Geometry: final body of the model. Coordinates: model frame, mm. Round coordinates to 2 decimals unless told otherwise and drop trailing zeros. Order: outer loops, then holes, each group sorted by start corner. A loop starts at its lowest first (then second) coordinate and runs counter-clockwise, first axis right, second up. Notation, with made-up numbers: (45, -13.75) -> (99, -13.75) arc R31 cw to (99, 12.25) -> close; hole circle Ø6 at (15.5, 54). An arc over 180 degrees is marked (long way). Put each result on its own line as item: value.
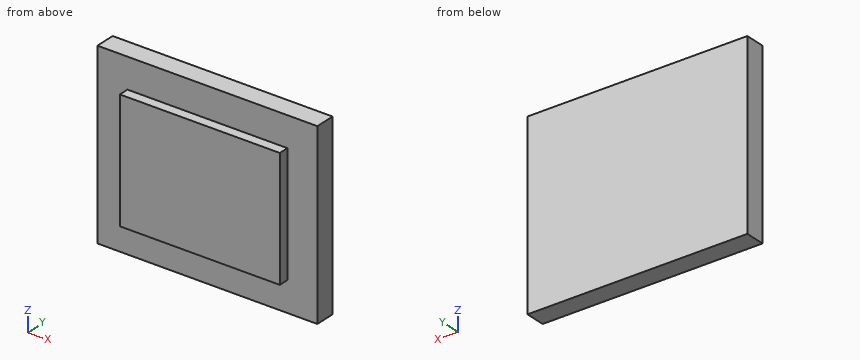
Solid Edge part; units mm, degrees
sketch "Sketch1" plane through (0, 0, 0) normal (0, -1, 0) x (1, 0, 0)
  line L0 (139.7, 114.3) -> (-139.7, 114.3)
  line L1 (-139.7, 114.3) -> (-139.7, -114.3)
  line L2 (-139.7, -114.3) -> (139.7, -114.3)
  line L3 (139.7, -114.3) -> (139.7, 114.3)
extrude "Protrusion1" add sketch "Sketch1" against normal blind 25.4
sketch "Sketch2" plane through (0, 0, 0) normal (0, -1, 0) x (1, 0, 0)
  line L0 (101.6, 76.2) -> (-101.6, 76.2)
  line L1 (-101.6, 76.2) -> (-101.6, -76.2)
  line L2 (-101.6, -76.2) -> (101.6, -76.2)
  line L3 (101.6, -76.2) -> (101.6, 76.2)
extrude "ExtrudedProtrusion_2" add sketch "Sketch2" along normal blind 12.7
1. Cut plane B-B on x = 26.5. Return loops of the section in (y, z).
Ans:
outline: (-12.7, -76.2) -> (0, -76.2) -> (0, -114.3) -> (25.4, -114.3) -> (25.4, 114.3) -> (0, 114.3) -> (0, 76.2) -> (-12.7, 76.2) -> close
2. Material intervals for probe 1 along Y at (x, z) = (14, 88.5); probe 2 along X at (y, z) = (-1.5, 31.5); probe 3 along Z at (x, y) = (-40, -4.5), sorted ascending.
Ans:
probe 1: 0 to 25.4
probe 2: -101.6 to 101.6
probe 3: -76.2 to 76.2
3. Contact query for flat-ended pins moving along their axis: P1, Ø10, axis at x = -11.5, y = -4, coming from the +Z side; P2, Ø5, axis at x = -20.5, y = -4.5, coming from the +Z side; P3, Ø10, axis at y = -7.5, z = 21, coming from the -X side; P4, Ø1, axis at x = 108, z = 81.5, coming from the -Y side. Output: stop coordinate, or through.
Ans:
P1: z = 114.3
P2: z = 76.2
P3: x = -101.6
P4: y = 0
4. Cut plane D-D on x = -121.5. Return loops of the section in (y, z), and give its area (3 significant figures).
Ans:
outline: (0, -114.3) -> (25.4, -114.3) -> (25.4, 114.3) -> (0, 114.3) -> close
area: 5,810 mm²
5. Cut plane A-A on z = 32. Return loops of the section in (x, y), and give its area (3 significant figures).
Ans:
outline: (-139.7, 0) -> (-101.6, 0) -> (-101.6, -12.7) -> (101.6, -12.7) -> (101.6, 0) -> (139.7, 0) -> (139.7, 25.4) -> (-139.7, 25.4) -> close
area: 9,680 mm²
6. Cut plane C-C on y = -5. Return loops of the section in (x, z).
Ans:
outline: (-101.6, -76.2) -> (101.6, -76.2) -> (101.6, 76.2) -> (-101.6, 76.2) -> close
